For this review, use the dimensioned drawing (mm, ordinates from the lowest corner) and the shaded views. A direction names the side the tool comes from. Coordinates: 2 decimals unless noted, no trailing zeros. Write each loop counter-clockwise with the first axis right and the second up, starting at its lowest first coordinate (ties: lowest second). Pieces come first, ordered by that corner, then holes. Notation, with made-up numbers: M 5.5,-35.5 L 57.5,-35.5 A16 ccw 57.5,-23.5 Z; hole C 52.25,57.25 d4. An arc over 180 degrees is marked long. Return JSON: item names as keys, results as strings.
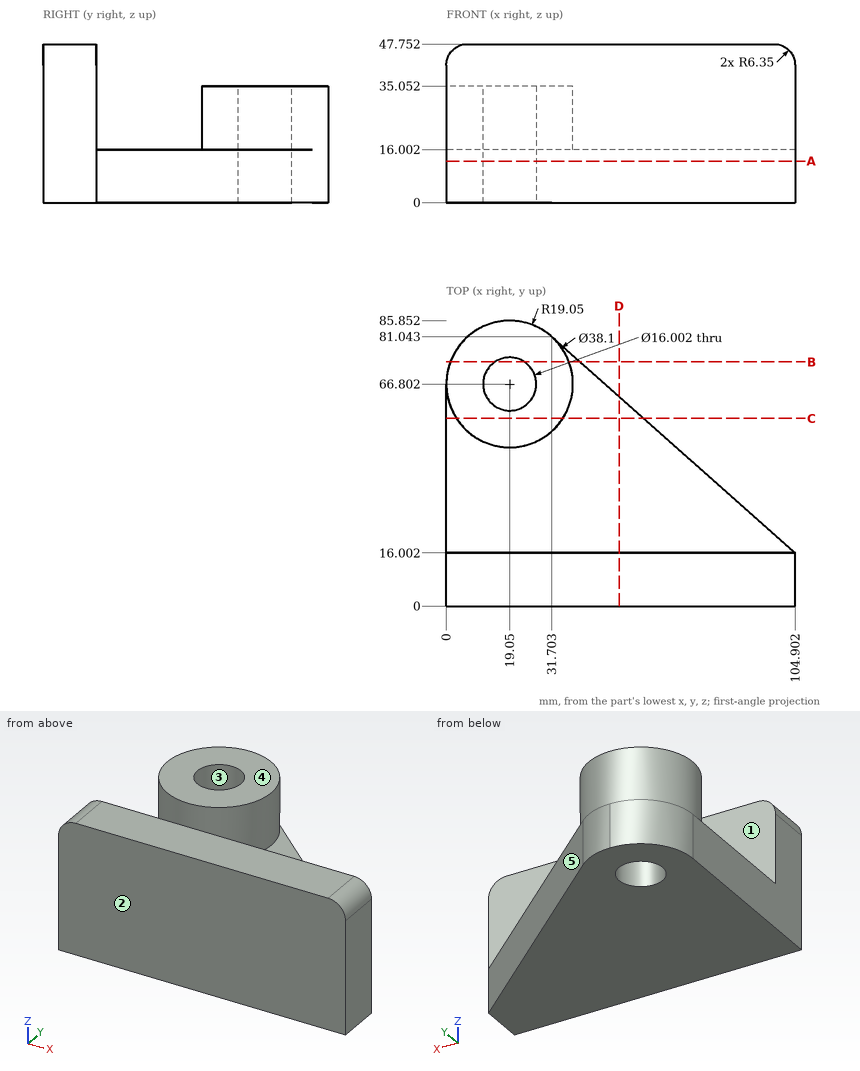
1. We need section C-C (y = 56.5). State the section outline as (x, z) points (1 decimal), plus the area to 3 significant figures.
Checks:
{"outline": "M 0,0 L 59.3,0 L 59.3,16 L 35.1,16 L 35.1,35.1 L 3,35.1 L 3,16 L 0,16 Z", "area": "1,560 mm2"}
2. We need section D-D (x = 52). State the section outline as (y, z) points, plus the area to 3 significant figures.
Checks:
{"outline": "M 0,0 L 63.01,0 L 63.01,16 L 16,16 L 16,47.75 L 0,47.75 Z", "area": "1,520 mm2"}
3. We need section A-A (z = 12.5). State the section outline as (x, y) points.
Checks:
{"outline": "M 0,0 L 104.9,0 L 104.9,16 L 31.7,81.04 A19.05 ccw 0,66.8 Z; hole C 19.05,66.8 d16"}
4. We need section B-B (y = 73.5). State the section outline as (x, z) points.
Checks:
{"outline": "M 1.22,0 L 14.67,0 L 14.67,35.05 L 1.22,35.05 Z; M 23.43,0 L 40.19,0 L 40.19,16 L 36.88,16 L 36.88,35.05 L 23.43,35.05 Z"}
5. Clearance check with flat-ended pins moving along their axes: pin 1 Ø10 at (x, y) = (59.5, 23) entering from +Z; pin 2 Ø21 at (x, y) = (19.05, 66.802) entering from +Z; pin 3 Ø12 at (y, z) = (70.5, 32) entering from -X; pin 4 Ø10 at (x, z) = (51.5, 17.5) entering from +Y. State where each tip first meets the part, or that it passes through.
Checks:
{"pin 1": "z = 16", "pin 2": "z = 35.05", "pin 3": "x = 0", "pin 4": "y = 67.69"}
6. For the marked faces 1 and 2, list the 3-axis set-ups (+Z, -Z, +X, -X, +Y, -Y) from which the entire face can be reached by the end or side of a thin tool; tool diameter is ignored.
Checks:
{"face 1": "+Z, +X, -X", "face 2": "+Z, -Z, +X, -X, -Y"}
7. Draft analysis for pull direction Y (two halves, no side actions). For the marked faces 3, 4 and 5, state which applies: +Y half, -Y half, draft (parallel to the pull), parting line (faces both ways), or undercut.
Checks:
{"face 3": "undercut", "face 4": "draft", "face 5": "+Y half"}
8. Wall thickness on L1, parallel to Y at x = 19.05, z = 24; L2, parallel to Y at x = 19, z = 11; L3, parallel to Z at x = 54, y = 58: over which ranges is each line inside the solid? List them lowest first. Write a range as from..to.
Checks:
{"L1": "0..16, 47.75..58.8, 74.8..85.85", "L2": "0..58.8, 74.8..85.85", "L3": "0..16"}
